The model under review builds one solid part; all positions refer to its coordinate system, in mm. A direction names the side the tool comes from. Round coordinates to 2 decimals unless told otherwise and drop trailing zeros. Order: outer loops, then holes, each group sorted by start corner. A loop starts at its lowest first (then second) coordinate and runs counter-clockwise, first axis right, second up.
```python
from build123d import *

# Parameters (mm, degrees)
SKETCH_1_R          = 7.5
SKETCH_1_R_2        = 0.9
SKETCH_1_R_3        = 4.45
EXTRUDE_1_DEPTH     = 1
SKETCH_2_R          = 5
EXTRUDE_2_DEPTH     = 4
SKETCH_3_R          = 4.45
CUT_EXTRUDE_1_DEPTH = 1
SKETCH_5_R          = 3
EXTRUDE_4_DEPTH     = 3
SKETCH_6_R          = 9
SKETCH_6_R_2        = 0.9
SKETCH_6_R_3        = 4.45
EXTRUDE_7_DEPTH     = 1
SKETCH_7_R          = 0.7
CUT_EXTRUDE_2_DEPTH = 10
SKETCH_8_R          = 9
SKETCH_8_R_2        = 7.6
CUT_EXTRUDE_3_DEPTH = 10


with BuildPart() as part:
    # 草图1 → 凸台-拉伸1 (new body)
    with BuildSketch(Plane.XY):
        Circle(SKETCH_1_R)
        with Locations((6, 0)):
            Circle(SKETCH_1_R_2, mode=Mode.SUBTRACT)
        with Locations((-3, -5.196152423)):
            Circle(SKETCH_1_R_2, mode=Mode.SUBTRACT)
        with Locations((-3, 5.196152423)):
            Circle(SKETCH_1_R_2, mode=Mode.SUBTRACT)
        Circle(SKETCH_1_R_3, mode=Mode.SUBTRACT)
    extrude(amount=EXTRUDE_1_DEPTH)

    # 草图2 → 凸台-拉伸2 (add)
    with BuildSketch(Plane.XY.offset(1)):
        Circle(SKETCH_2_R)
    extrude(amount=EXTRUDE_2_DEPTH)

    # 草图3 → 切除-拉伸1 (cut)
    with BuildSketch(Plane(origin=(0, 0, 1), x_dir=(-1, 0, 0), z_dir=(0, 0, -1))):
        Circle(SKETCH_3_R)
    extrude(amount=-CUT_EXTRUDE_1_DEPTH, mode=Mode.SUBTRACT)

    # 草图5 → 凸台-拉伸4 (add)
    with BuildSketch(Plane.XY.offset(5)):
        with Locations((0.5, 0)):
            Circle(SKETCH_5_R)
    extrude(amount=EXTRUDE_4_DEPTH)

    # 草图6 → 凸台-拉伸7 (add)
    with BuildSketch(Plane.XY.offset(1)):
        Circle(SKETCH_6_R)
        with Locations((6, 0)):
            Circle(SKETCH_6_R_2, mode=Mode.SUBTRACT)
        with Locations((-3, 5.196152423)):
            Circle(SKETCH_6_R_2, mode=Mode.SUBTRACT)
        with Locations((-3, -5.196152423)):
            Circle(SKETCH_6_R_2, mode=Mode.SUBTRACT)
        Circle(SKETCH_6_R_3, mode=Mode.SUBTRACT)
    extrude(amount=-EXTRUDE_7_DEPTH)

    # 草图7 → 切除-拉伸2 (cut)
    with BuildSketch(Plane.XY.offset(8)):
        with Locations((-0.5, 1.3)):
            Circle(SKETCH_7_R)
        with Locations((-0.5, -1.3)):
            Circle(SKETCH_7_R)
    extrude(amount=-CUT_EXTRUDE_2_DEPTH, mode=Mode.SUBTRACT)

    # 草图8 → 切除-拉伸3 (cut)
    with BuildSketch(Plane.XY.offset(1)):
        Circle(SKETCH_8_R)
        Circle(SKETCH_8_R_2, mode=Mode.SUBTRACT)
    extrude(amount=-CUT_EXTRUDE_3_DEPTH, mode=Mode.SUBTRACT)


solid = part.part
```
(1) Consider section B-B (x = -3). Write out the cut boundary in (y, z).
Data:
outline: (-6.98, 0) - (-6.1, 0) - (-6.1, 1) - (-6.98, 1) - close; (-4.3, 0) - (-3.29, 0) - (-3.29, 2) - (3.29, 2) - (3.29, 0) - (4.3, 0) - (4.3, 1) - (4, 1) - (4, 5) - (-4, 5) - (-4, 1) - (-4.3, 1) - close; (6.1, 0) - (6.98, 0) - (6.98, 1) - (6.1, 1) - close
(2) For faces 1 (the cylindrical face through (-1.08, -4.88, 2.97)), 2 (the flat face through (0, 0, 2)), 3 (the cylindrical face through (-2.17, 4.85, 0.49)), list the 3-axis set-ups (+Z, -Z, +X, -X, +Y, -Y) from which the entire face can be reached by the end or side of a thin tool; tool diameter is ignored.
Data:
face 1: +Z
face 2: -Z
face 3: +Z, -Z
(3) Insertion check: pin 1 (2 mm diameter, centred on x = -3, y = -5.2, fed in from -Z); pin 2 (1 mm diameter, centred on y = 0, z = 4, fed in from -X); pin 3 (1.1 mm diameter, centred on x = -0.5, y = -1.3, fed in from +Z); pin 4 (1.5 mm diameter, centred on x = -3.5, z = 4, fed in from -Y). Each pin has a flat end and moves straight along its axis. Give the tip position at first contact, or say it passes through.
Data:
pin 1: stops at z = 0
pin 2: stops at x = -5
pin 3: passes through
pin 4: stops at y = -4.18
(4) Consider section D-D (z = 4). Write out the cut boundary in (x, y), and give its area (3 significant figures).
Data:
outline: circle Ø10 at (0, 0); hole circle Ø1.4 at (-0.5, -1.3); hole circle Ø1.4 at (-0.5, 1.3)
area: 75.5 mm2
(5) Consider section A-A (y = 0). Write out the cut boundary in (x, z).
Data:
outline: (-7.6, 0) - (-4.45, 0) - (-4.45, 2) - (4.45, 2) - (4.45, 0) - (5.1, 0) - (5.1, 1) - (5, 1) - (5, 5) - (3.5, 5) - (3.5, 8) - (-2.5, 8) - (-2.5, 5) - (-5, 5) - (-5, 1) - (-7.6, 1) - close; (6.9, 0) - (7.6, 0) - (7.6, 1) - (6.9, 1) - close
(6) To check wall thickness, follow probe 1 along Y at (x, z) = (-0.5, 4); probe 2 along Y at (x, z) = (-3, 0.5); probe 3 along Z at (x, y) = (-5.5, 2). State the ranges of each line that lie inside material, in increasing order.
Data:
probe 1: y = -4.97 to -2, -0.6 to 0.6, 2 to 4.97
probe 2: y = -6.98 to -6.1, -4.3 to -3.29, 3.29 to 4.3, 6.1 to 6.98
probe 3: z = 0 to 1
(7) Consider section C-C (x = 6). Write out the cut boundary in (y, z), and give its area (3 significant figures).
Data:
outline: (-4.66, 0) - (-0.9, 0) - (-0.9, 1) - (-4.66, 1) - close; (0.9, 0) - (4.66, 0) - (4.66, 1) - (0.9, 1) - close
area: 7.53 mm2
(8) Draft analysis for pull direction X (two halves, no side actions). For faces 4 (the cylindrical face through (-7.593, 0.334, 0.507)), 5 (the cylindrical face through (5.1, 0, 0.5)), 6 (the flat face through (-2, -2, 5)), state which applies: pulls with the +X half, pulls with the -X half, needs draft (parallel to the pull), parting line crosses it, or undercut.
Data:
face 4: parting line crosses it
face 5: undercut
face 6: needs draft
